from build123d import *

# Parameters (mm, degrees)
SKETCH1_R           = 2
BOSS_EXTRUDE1_DEPTH = 2
BOSS_EXTRUDE2_START = 2
BOSS_EXTRUDE2_DEPTH = 3
SKETCH3_R           = 2
BOSS_EXTRUDE3_DEPTH = 2
BOSS_EXTRUDE4_START = 2
BOSS_EXTRUDE4_DEPTH = 3
SKETCH4_W           = 44.205836774
SKETCH4_H           = 30
SKETCH4_R           = 2
BOSS_EXTRUDE5_DEPTH = 2
BOSS_EXTRUDE6_START = 2
SKETCH4_4_W         = 44.205836774
SKETCH4_4_H         = 30
BOSS_EXTRUDE6_DEPTH = 3
CUT_EXTRUDE1_START  = 2
SKETCH3_5_R         = 2
CUT_EXTRUDE1_DEPTH  = 10


with BuildPart() as part:
    # Sketch1 → Boss-Extrude1 (new body)
    # profile 1 of 3: a face of its own
    with BuildSketch(Plane.XY):
        Polygon((15.156849888, -300.73734036), (-27.167723767, -320.473613183), (-39.846271619, -293.284379572), (2.478302036, -273.548106749), align=None)
        Polygon((-22.447739873, -291.889732471), (-24.410730789, -295.289732471), (-22.447739873, -298.689732471), (-18.521758043, -298.689732471), (-16.558767128, -295.289732471), (-18.521758043, -291.889732471), align=None, mode=Mode.SUBTRACT)
        Polygon((-4.321584133, -283.437367237), (-6.284575048, -286.837367237), (-4.321584133, -290.237367237), (-0.395602302, -290.237367237), (1.567388613, -286.837367237), (-0.395602302, -283.437367237), align=None, mode=Mode.SUBTRACT)
    # profile 2 of 3: a face of its own
    with BuildSketch(Plane.XY):
        Polygon((-0.395602302, -283.437367237), (-4.321584133, -283.437367237), (-6.284575048, -286.837367237), (-4.321584133, -290.237367237), (-0.395602302, -290.237367237), (1.567388613, -286.837367237), align=None)
        with Locations((-2.358593217, -286.837367237)):
            Circle(SKETCH1_R, mode=Mode.SUBTRACT)
    # profile 3 of 3: a face of its own
    with BuildSketch(Plane.XY):
        Polygon((-18.521758043, -291.889732471), (-22.447739873, -291.889732471), (-24.410730789, -295.289732471), (-22.447739873, -298.689732471), (-18.521758043, -298.689732471), (-16.558767128, -295.289732471), align=None)
        with Locations((-20.484748958, -295.289732471)):
            Circle(SKETCH1_R, mode=Mode.SUBTRACT)
    extrude(amount=BOSS_EXTRUDE1_DEPTH)

    # Sketch1<3> → Boss-Extrude2 (add)
    with BuildSketch(Plane.XY.offset(BOSS_EXTRUDE2_START)):
        Polygon((15.156849888, -300.73734036), (-27.167723767, -320.473613183), (-39.846271619, -293.284379572), (2.478302036, -273.548106749), align=None)
        Polygon((-22.447739873, -291.889732471), (-24.410730789, -295.289732471), (-22.447739873, -298.689732471), (-18.521758043, -298.689732471), (-16.558767128, -295.289732471), (-18.521758043, -291.889732471), align=None, mode=Mode.SUBTRACT)
        Polygon((-4.321584133, -283.437367237), (-6.284575048, -286.837367237), (-4.321584133, -290.237367237), (-0.395602302, -290.237367237), (1.567388613, -286.837367237), (-0.395602302, -283.437367237), align=None, mode=Mode.SUBTRACT)
    extrude(amount=BOSS_EXTRUDE2_DEPTH)

    # Sketch3 → Boss-Extrude3 (add)
    # profile 1 of 3: a face of its own
    with BuildSketch(Plane(origin=(117.8961915, -252.829198573, 0), x_dir=(0.9063077870366509, 0.42261826174069744, 0), z_dir=(-0.42261826174069744, 0.9063077870366509, 0))):
        Polygon((-113.360320943, 0), (-160.060320943, 0), (-160.060320943, -5), (-160.060320943, -49.205836774), (-113.360320943, -5), align=None)
        Polygon((-149.353719225, -30.482796069), (-149.353719225, -26.556814238), (-152.753719225, -24.593823323), (-156.153719225, -26.556814238), (-156.153719225, -30.482796069), (-152.753719225, -32.445786984), align=None, mode=Mode.SUBTRACT)
        Polygon((-128.14051579, -5.343610803), (-131.54051579, -3.380619887), (-134.94051579, -5.343610803), (-134.94051579, -9.269592633), (-131.54051579, -11.232583548), (-128.14051579, -9.269592633), align=None, mode=Mode.SUBTRACT)
    # profile 2 of 3: a face of its own
    with BuildSketch(Plane(origin=(117.8961915, -252.829198573, 0), x_dir=(0.9063077870366509, 0.42261826174069744, 0), z_dir=(-0.42261826174069744, 0.9063077870366509, 0))):
        Polygon((-128.14051579, -5.343610803), (-128.735667158, -5), (-134.345364422, -5), (-134.94051579, -5.343610803), (-134.94051579, -9.269592633), (-131.54051579, -11.232583548), (-128.14051579, -9.269592633), align=None)
        with Locations(Location((-131.54051579, -7.306601718, 0), (0, 0, 180))):
            Circle(SKETCH3_R, mode=Mode.SUBTRACT)
    # profile 3 of 3: a face of its own
    with BuildSketch(Plane(origin=(117.8961915, -252.829198573, 0), x_dir=(0.9063077870366509, 0.42261826174069744, 0), z_dir=(-0.42261826174069744, 0.9063077870366509, 0))):
        Polygon((-149.353719225, -30.482796069), (-149.353719225, -26.556814238), (-152.753719225, -24.593823323), (-156.153719225, -26.556814238), (-156.153719225, -30.482796069), (-152.753719225, -32.445786984), align=None)
        with Locations(Location((-152.753719225, -28.519805153, 0), (0, 0, 180))):
            Circle(SKETCH3_R, mode=Mode.SUBTRACT)
    extrude(amount=BOSS_EXTRUDE3_DEPTH)

    # Sketch3<4> → Boss-Extrude4 (add)
    with BuildSketch(Plane(origin=(117.8961915, -252.829198573, 0), x_dir=(0.9063077870366509, 0.42261826174069744, 0), z_dir=(-0.42261826174069744, 0.9063077870366509, 0)).offset(BOSS_EXTRUDE4_START)):
        Polygon((-113.360320943, 0), (-160.060320943, 0), (-160.060320943, -5), (-160.060320943, -49.205836774), (-113.360320943, -5), align=None)
        Polygon((-149.353719225, -30.482796069), (-149.353719225, -26.556814238), (-152.753719225, -24.593823323), (-156.153719225, -26.556814238), (-156.153719225, -30.482796069), (-152.753719225, -32.445786984), align=None, mode=Mode.SUBTRACT)
        Polygon((-128.14051579, -5.343610803), (-131.54051579, -3.380619887), (-134.94051579, -5.343610803), (-134.94051579, -9.269592633), (-131.54051579, -11.232583548), (-128.14051579, -9.269592633), align=None, mode=Mode.SUBTRACT)
    extrude(amount=BOSS_EXTRUDE4_DEPTH)

    # Sketch4 → Boss-Extrude5 (add)
    # profile 1 of 3: a face of its own
    with BuildSketch(Plane(origin=(-145.063915266, -67.644414611, 0), x_dir=(0, 0, -1), z_dir=(0.9063077870366509, 0.42261826174069744, 1.6586764924388181e-15))):
        with Locations((-27.102918387, -263.966154974)):
            Rectangle(SKETCH4_W, SKETCH4_H)
        Polygon((-31.962990915, -272.366154974), (-33.92598183, -268.966154974), (-31.962990915, -265.566154974), (-28.037009085, -265.566154974), (-26.07401817, -268.966154974), (-28.037009085, -272.366154974), align=None, mode=Mode.SUBTRACT)
        Polygon((-11.962990915, -272.366154974), (-13.92598183, -268.966154974), (-11.962990915, -265.566154974), (-8.037009085, -265.566154974), (-6.07401817, -268.966154974), (-8.037009085, -272.366154974), align=None, mode=Mode.SUBTRACT)
    # profile 2 of 3: a face of its own
    with BuildSketch(Plane(origin=(-145.063915266, -67.644414611, 0), x_dir=(0, 0, -1), z_dir=(0.9063077870366509, 0.42261826174069744, 1.6586764924388181e-15))):
        Polygon((-28.037009085, -265.566154974), (-31.962990915, -265.566154974), (-33.92598183, -268.966154974), (-31.962990915, -272.366154974), (-28.037009085, -272.366154974), (-26.07401817, -268.966154974), align=None)
        with Locations(Location((-30, -268.966154974, 0), (0, 0, 90))):
            Circle(SKETCH4_R, mode=Mode.SUBTRACT)
    # profile 3 of 3: a face of its own
    with BuildSketch(Plane(origin=(-145.063915266, -67.644414611, 0), x_dir=(0, 0, -1), z_dir=(0.9063077870366509, 0.42261826174069744, 1.6586764924388181e-15))):
        Polygon((-8.037009085, -265.566154974), (-11.962990915, -265.566154974), (-13.92598183, -268.966154974), (-11.962990915, -272.366154974), (-8.037009085, -272.366154974), (-6.07401817, -268.966154974), align=None)
        with Locations(Location((-10, -268.966154974, 0), (0, 0, 90))):
            Circle(SKETCH4_R, mode=Mode.SUBTRACT)
    extrude(amount=BOSS_EXTRUDE5_DEPTH)

    # Sketch4<4> → Boss-Extrude6 (add)
    with BuildSketch(Plane(origin=(-145.063915266, -67.644414611, 0), x_dir=(0, 0, -1), z_dir=(0.9063077870366509, 0.42261826174069744, 1.6586764924388181e-15)).offset(BOSS_EXTRUDE6_START)):
        with Locations((-27.102918387, -263.966154974)):
            Rectangle(SKETCH4_4_W, SKETCH4_4_H)
        Polygon((-31.962990915, -272.366154974), (-33.92598183, -268.966154974), (-31.962990915, -265.566154974), (-28.037009085, -265.566154974), (-26.07401817, -268.966154974), (-28.037009085, -272.366154974), align=None, mode=Mode.SUBTRACT)
        Polygon((-11.962990915, -272.366154974), (-13.92598183, -268.966154974), (-11.962990915, -265.566154974), (-8.037009085, -265.566154974), (-6.07401817, -268.966154974), (-8.037009085, -272.366154974), align=None, mode=Mode.SUBTRACT)
    extrude(amount=BOSS_EXTRUDE6_DEPTH)

    # Sketch3<5> → Cut-Extrude1 (cut)
    # profile 1 of 2: a face of its own
    with BuildSketch(Plane(origin=(117.8961915, -252.829198573, 0), x_dir=(0.9063077870366509, 0.42261826174069744, 0), z_dir=(-0.42261826174069744, 0.9063077870366509, 0)).offset(CUT_EXTRUDE1_START)):
        Polygon((-128.14051579, -5.343610803), (-131.54051579, -3.380619887), (-134.94051579, -5.343610803), (-134.94051579, -9.269592633), (-131.54051579, -11.232583548), (-128.14051579, -9.269592633), align=None)
        with Locations(Location((-131.54051579, -7.306601718, 0), (0, 0, 180))):
            Circle(SKETCH3_5_R, mode=Mode.SUBTRACT)
    # profile 2 of 2: a face of its own
    with BuildSketch(Plane(origin=(117.8961915, -252.829198573, 0), x_dir=(0.9063077870366509, 0.42261826174069744, 0), z_dir=(-0.42261826174069744, 0.9063077870366509, 0)).offset(CUT_EXTRUDE1_START)):
        Polygon((-149.353719225, -30.482796069), (-149.353719225, -26.556814238), (-152.753719225, -24.593823323), (-156.153719225, -26.556814238), (-156.153719225, -30.482796069), (-152.753719225, -32.445786984), align=None)
        with Locations(Location((-152.753719225, -28.519805153, 0), (0, 0, 180))):
            Circle(SKETCH3_5_R, mode=Mode.SUBTRACT)
    extrude(amount=CUT_EXTRUDE1_DEPTH, mode=Mode.SUBTRACT)


solid = part.part
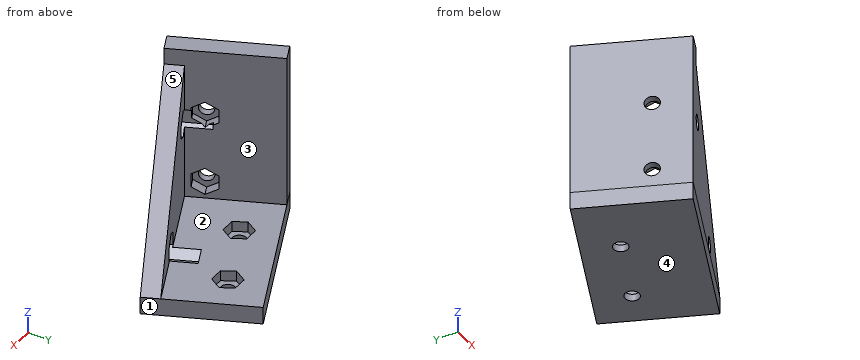
Read the model definition and answer for the solid it produces. Units are mm, in the model's axes. Face numbers are marked on the shaded views. A direction names the side the tool comes from. Coordinates: 2 decimals unless noted, no trailing zeros. Loops run counter-clockwise (first coordinate to the right, second up) from the corner with the lowest first, then second, coordinate; pieces in that order, holes last. Notation, with made-up numbers: (60.5, 50) - (95.5, 50) arc R25 cw to (95.5, 83) - close; hole circle Ø5 at (9, 43). An arc over 180 degrees is marked (long way). Answer in a Markdown table with one row per item.
Q1. Given P1, Ø1.5, axis at y = -311.5, z = 5.5, coming from the -X side; P2, Ø3, axis at x = -7, z = 28, coming from the -Y side; P3, Ø1.5, axis at x = -21, z = 4, coming from the -Y side; P4, Ø8, axis at x = -2.5, y = -284.5, coming from the -Z side, each flat-ended and moving along its own axis, determine where each tip first touches the part or whether it passes through.
Here are the results:
| item | result |
|---|---|
| P1 | stops at x = -31.7 |
| P2 | stops at y = -311.77 |
| P3 | stops at y = -317.95 |
| P4 | stops at z = 0 |
Q2. For the marked faces 1 and 2, determine the directions among +Z, -Z, +X, -X, +Y, -Y from which every point of the face is accessible in a straight line to the end or side of a thin tool.
Here are the results:
| item | result |
|---|---|
| face 1 | +Z, -Z, +X, +Y |
| face 2 | +Z, +Y |
Q3. The mould has two halves that part along X. Classify the marked faces 3, 4 and 5: pulls with the +X half, pulls with the -X half, needs draft (parallel to the pull), parting line crosses it, or undercut.
Here are the results:
| item | result |
|---|---|
| face 3 | undercut |
| face 4 | needs draft |
| face 5 | pulls with the +X half |
Q4. Find section C-C on y = -281.5. Write down the section's boundary in (x, z).
Here are the results:
| item | result |
|---|---|
| outline | (-14.57, 0) - (6.19, 0) - (6.19, 5) - (-14.57, 5) - close |
Q5. Straight lines are drawn through the part: line 1 along Z through (x, y) = (-28, -307); line 2 along Z through (x, y) = (-27.5, -295.5); line 3 along Y through (x, z) = (-19, 28.5). For each, find the intervals that lie inside material, in ascending order. Write a range as [from, to].
Here are the results:
| item | result |
|---|---|
| line 1 | z = [0, 7.55], [12.45, 27.55], [32.45, 49.21] |
| line 2 | z = [0, 5] |
| line 3 | y = [-315.97, -314.46], [-312.66, -311.15] |
Q6. Find section A-A on z = 35. Write down the section's boundary in (x, y), plus the area to 3 significant figures.
Here are the results:
| item | result |
|---|---|
| outline | (-39.85, -293.28) - (-27.17, -320.47) - (-13.57, -314.13) - (-15.68, -309.6) - (-24.75, -313.83) - (-35.31, -291.17) - close |
| area | 200 mm^2 |
Q7. Find section D-D on z = 17.5. Write down the section's boundary in (x, y).
Here are the results:
| item | result |
|---|---|
| outline | (-39.85, -293.28) - (-27.17, -320.47) - (3.19, -306.32) - (1.08, -301.79) - (-24.75, -313.83) - (-35.31, -291.17) - close |
Q8. Find section B-B on x = 4. Write down the section's boundary in (y, z).
Here are the results:
| item | result |
|---|---|
| outline | (-305.94, 0) - (-276.81, 0) - (-276.81, 5) - (-300.42, 5) - (-300.42, 14.45) - (-305.94, 16.65) - close |
